Read the model definition and answer for the solid it produces. Units are mm, in the model's axes. Face numbers are marked on the shaded views. A direction names the side the tool comes from. Round coordinates to 2 decimals unless told otherwise and drop trailing zeros. Order: outer loops, then holes, each group sorted by start corner. A loop starts at its lowest first (then second) coordinate and runs counter-clockwise, first axis right, second up. Notation, with made-up numbers: M 68,-22 L 78,-22 A18 cw 78,-10 Z; hole C 74.5,-13.5 d8. An arc over 180 degrees is marked long. Answer as CSV lines item,"result".
```python
from build123d import *

# Parameters (mm, degrees)
PAD_DEPTH    = 10
POCKET_DEPTH = 10.001


with BuildPart() as part:
    # Sketch → Pad (new body)
    with BuildSketch(Plane.XY):
        Polygon((-41.231688, -29.660868), (41.009132, -29.660868), (34.035849, -10.50193), (19.169409, -5.090988), (40.721873, 2.753467), (40.721873, 19.774112), (23.629803, 19.774112), (17.888071, 35.549391), (9.458496, 12.389326), (-48.365379, 22.585235), (-48.365379, 4.987422), (-51.376506, -12.089527), align=None)
    extrude(amount=PAD_DEPTH)

    # Sketch001 (on Face14 of Pad) → Pocket (cut, through all)
    with BuildSketch(Plane.XY.offset(10)):
        Polygon((-7.902639, -14.299959), (-13.287209, -4.97361), (-7.902639, 4.35274), (-18.67178, 4.35274), (-24.05635, 13.679089), (-29.440921, 4.35274), (-40.210062, 4.35274), (-34.825491, -4.97361), (-40.210062, -14.299959), (-29.440921, -14.299959), (-24.05635, -23.626309), (-18.67178, -14.299959), align=None)
    extrude(amount=-POCKET_DEPTH, mode=Mode.SUBTRACT)


solid = part.part
```
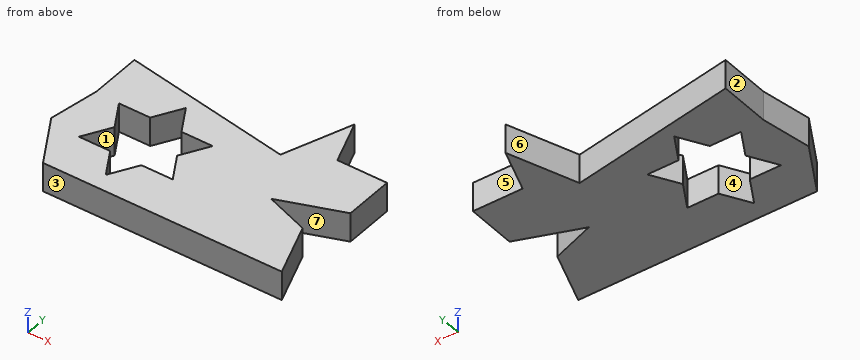
Item 1: Find the intervals of material crossed by probe 1 along Y at (x, z) = (-13, 8.5); probe 2 along Y at (x, z) = (-39.5, 4); probe 3 along Y at (x, z) = (30, 2.75), in increasing order. Write a range as [from, to].
Ans:
probe 1,"[-29.66, -14.3], [-5.47, -4.48], [4.35, 16.35]"
probe 2,"[-29.66, -14.3], [-13.07, 3.12], [4.35, 21.02]"
probe 3,"[-29.66, -9.03], [-1.15, 19.77]"
Item 2: A tool of negligible diameter and unlimited length cuts with its end or side. For the marked faces 4, 5, 6 and 7, from which of +Z, -Z, +X, -X, +Y, -Y can it reach the whole face along a straight path? Write none if from no direction.
Ans:
face 4,"+Z, -Z"
face 5,"+Z, -Z, +X, +Y"
face 6,"+Z, -Z, +Y"
face 7,"+Z, -Z, +X"
Item 3: A cutting plane is placed at B-B, the plane x = 26.5. Determine the outline of the cut face in (y, z), and give its area (3 significant figures).
Ans:
outline,"M -29.66,0 L -7.76,0 L -7.76,10 L -29.66,10 Z; M -2.42,0 L 19.77,0 L 19.77,10 L -2.42,10 Z"
area,"441 mm2"
Item 4: A cutting plane is placed at A-A, the plane y = -19. Determine the outline of the cut face in (x, z), and give its area (3 significant figures).
Ans:
outline,"M -47.39,0 L -26.73,0 L -26.73,10 L -47.39,10 Z; M -21.39,0 L 37.13,0 L 37.13,10 L -21.39,10 Z"
area,"792 mm2"
Item 5: A cutting plane is placed at D-D, the plane x = -11.5. Determine the outline of the cut face in (y, z), and give its area (3 significant figures).
Ans:
outline,"M -29.66,0 L -14.3,0 L -14.3,10 L -29.66,10 Z; M -8.07,0 L -1.88,0 L -1.88,10 L -8.07,10 Z; M 4.35,0 L 16.08,0 L 16.08,10 L 4.35,10 Z"
area,"333 mm2"
Item 6: Determine the mould class of the marked faces 1, 2 and 3 for opening direction X: +X half, -X half, draft (parallel to the pull), parting line (faces both ways), or undercut.
Ans:
face 1,"undercut"
face 2,"-X half"
face 3,"draft"
Item 7: A cutting plane is placed at C-C, the plane z = 3.25. Determine the outline of the cut face in (x, y), and give its area (3 significant figures).
Ans:
outline,"M -51.38,-12.09 L -41.23,-29.66 L 41.01,-29.66 L 34.04,-10.5 L 19.17,-5.09 L 40.72,2.75 L 40.72,19.77 L 23.63,19.77 L 17.89,35.55 L 9.46,12.39 L -48.37,22.59 L -48.37,4.99 Z; hole M -40.21,-14.3 L -29.44,-14.3 L -24.06,-23.63 L -18.67,-14.3 L -7.9,-14.3 L -13.29,-4.97 L -7.9,4.35 L -18.67,4.35 L -24.06,13.68 L -29.44,4.35 L -40.21,4.35 L -34.83,-4.97 Z"
area,"3,520 mm2"
Item 8: Flat-ended cylindrical pins translate along their axes: pin 1 (3 mm diameter, centred on x = -13, z = 5, fed in from +Y); pin 2 (1.5 mm diameter, centred on x = -14.5, y = 10.5, fed in from -Z); pin 3 (5 mm diameter, centred on x = 26.5, z = 8.5, fed in from +Y); pin 4 (5 mm diameter, centred on y = 10, z = 3.5, fed in from +X). Find the tip coordinate at first contact, or state that the pin passes through.
Ans:
pin 1,"y = 16.61"
pin 2,"z = 0"
pin 3,"y = 19.77"
pin 4,"x = 40.72"
